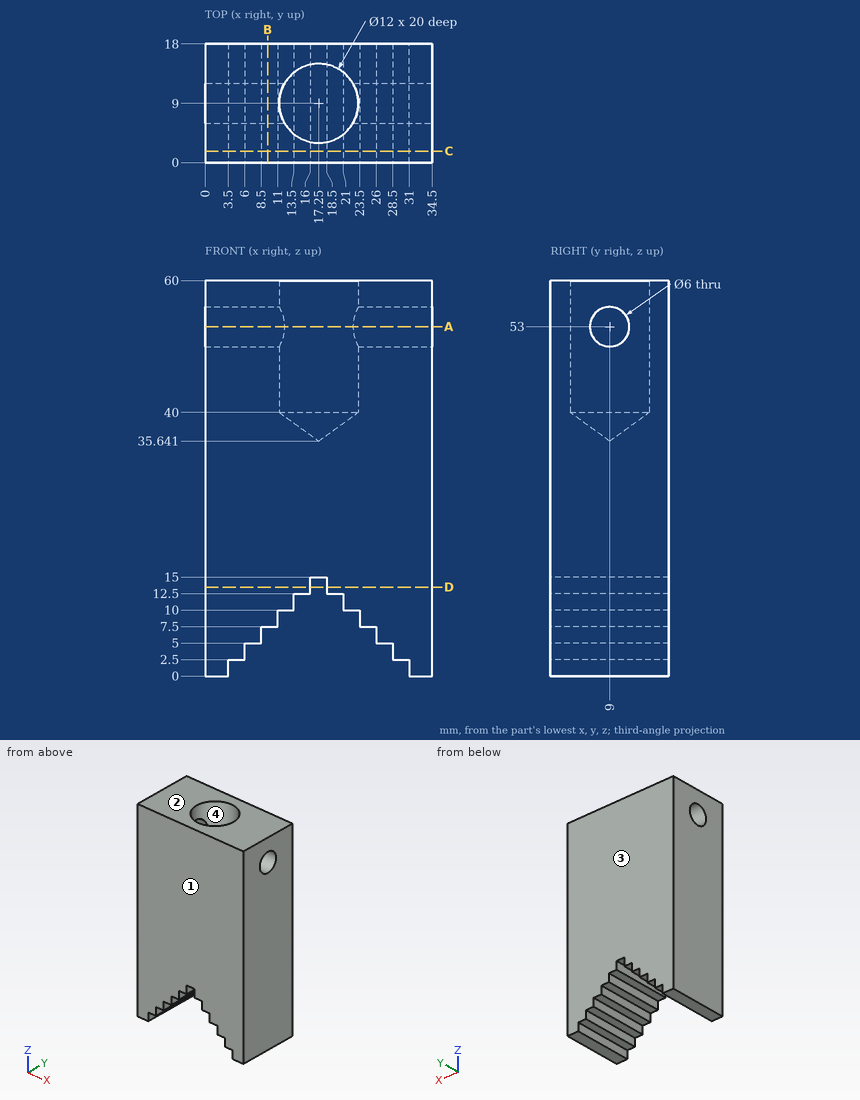
Input: dimensioned drawing with shaded views. Units: mm. Origin: part minimum x, y, z. Coordinates: 2 decimals unless noted, no trailing zeros. Order: outer loops, then holes, each group sorted by start corner. A loop starts at its lowest first (then second) coordinate and runs counter-clockwise, first axis right, second up.
Item 1: Contact query for flat-ended pins moving along their axis: P1, Ø0.8, axis at x = 24.5, y = 7.5, coming from the -Z side; P2, Ø1.2, axis at x = 4.5, y = 4.5, coming from the -Z side. Output: stop coordinate, or through.
Answer:
P1: stops at z = 7.5
P2: stops at z = 2.5
Item 2: Section query B-B (x = 9.5). Output: boundary loops of the cut face in (y, z), then the cut area to 3 significant figures.
Answer:
outline: (0, 7.5) - (18, 7.5) - (18, 60) - (0, 60) - close; hole circle Ø6 at (9, 53)
area: 917 mm2
Item 3: Material intervals for line 1 along X through (y, z) = (15.25, 3); line 2 along Z through (x, y) = (6.5, 9); line 3 along Y through (x, z) = (4, 53), sorted ascending.
Answer:
line 1: x = 0 to 6, 28.5 to 34.5
line 2: z = 5 to 50, 56 to 60
line 3: y = 0 to 6, 12 to 18
Item 4: Section query D-D (z = 13.5). Output: boundary loops of the cut face in (x, y), then the cut area to 3 significant figures.
Answer:
outline: (0, 0) - (16, 0) - (16, 18) - (0, 18) - close; (18.5, 0) - (34.5, 0) - (34.5, 18) - (18.5, 18) - close
area: 576 mm2
Item 5: Section query C-C (y = 1.75). Output: boundary loops of the cut face in (x, z).
Answer:
outline: (0, 0) - (3.5, 0) - (3.5, 2.5) - (6, 2.5) - (6, 5) - (8.5, 5) - (8.5, 7.5) - (11, 7.5) - (11, 10) - (13.5, 10) - (13.5, 12.5) - (16, 12.5) - (16, 15) - (18.5, 15) - (18.5, 12.5) - (21, 12.5) - (21, 10) - (23.5, 10) - (23.5, 7.5) - (26, 7.5) - (26, 5) - (28.5, 5) - (28.5, 2.5) - (31, 2.5) - (31, 0) - (34.5, 0) - (34.5, 60) - (0, 60) - close
Item 6: Draft query along Y for the marked faces 1, 2, 3 and 4. Return one class per face: released by +Y, released by -Y, zero draft, split by the parting line, or undercut.
Answer:
face 1: released by -Y
face 2: zero draft
face 3: released by +Y
face 4: undercut
Item 7: Section query A-A (z = 53). Output: boundary loops of the cut face in (x, y), then the cut area to 3 significant figures.
Answer:
outline: (0, 0) - (34.5, 0) - (34.5, 6) - (22.45, 6) arc R6 cw to (12.05, 6) - (0, 6) - close; (0, 12) - (12.05, 12) arc R6 cw to (22.45, 12) - (34.5, 12) - (34.5, 18) - (0, 18) - close
area: 370 mm2
